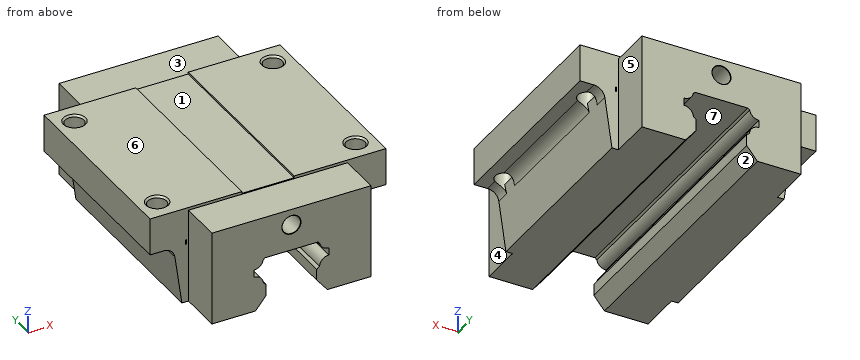
from build123d import *

# Parameters (mm, degrees)
SKIZZE1_W                       = 44
SKIZZE1_H                       = 51.3
AUFSATZ_LINEAR_AUSTRAGEN1_DEPTH = 26
SKIZZE2_W                       = 0.25
SKIZZE2_H                       = 17.25
SCHNITT_LINEAR_AUSTRAGEN1_DEPTH = 64.369472146
SKIZZE3_W                       = 14
SKIZZE3_H                       = 0.5
SCHNITT_LINEAR_AUSTRAGEN2_DEPTH = 64.369472146
SKIZZE4_W                       = 0.25
SKIZZE4_H                       = 17.25
SCHNITT_LINEAR_AUSTRAGEN3_DEPTH = 51.3
SKIZZE5_W                       = 42.5
SKIZZE5_H                       = 25.25
AUFSATZ_LINEAR_AUSTRAGEN2_DEPTH = 11.35
SKIZZE6_W                       = 42.5
SKIZZE6_H                       = 25.25
AUFSATZ_LINEAR_AUSTRAGEN3_DEPTH = 11.35
SKIZZE15_W                      = 9.5
SKIZZE15_H                      = 51.3
AUFSATZ_LINEAR_AUSTRAGEN5_DEPTH = 10
SCHNITT_LINEAR_AUSTRAGEN4_DEPTH = 86.838511171
BOHRUNG1_D                      = 4.917
BOHRUNG1_DEPTH                  = 15
BOHRUNG1_TIP                    = 1.477215832
BOHRUNG2_D                      = 4.917
BOHRUNG2_DEPTH                  = 15
BOHRUNG2_TIP                    = 1.477215832
M6_GEWINDEBOHRUNG1_D            = 5
M6_GEWINDEBOHRUNG1_DEPTH        = 17
M6_GEWINDEBOHRUNG1_TIP          = 1.502151548
FASE1_SIZE                      = 0.483
FASE2_SIZE                      = 0.448979592
FASE3_SIZE                      = 0.0915
FASE4_SIZE                      = 0.448979592
AUFSATZ_LINEAR_START            = -51.3
AUFSATZ_LINEAR_AUSTRAGEN6_DEPTH = 51.3
VERRUNDUNG1_R                   = 3


with BuildPart() as part:
    # Skizze1 → Aufsatz-Linear austragen1 (new body)
    with BuildSketch(Plane(origin=(0, 0, 4), x_dir=(-1, 0, 0), z_dir=(0, 0, -1))):
        Rectangle(SKIZZE1_W, SKIZZE1_H)
    extrude(amount=-AUFSATZ_LINEAR_AUSTRAGEN1_DEPTH)

    # Skizze2 → Schnitt-Linear austragen1 (cut, through all)
    with BuildSketch(Plane.XZ.offset(25.65)):
        with Locations((-21.875, 12.625)):
            Rectangle(SKIZZE2_W, SKIZZE2_H)
    extrude(amount=-SCHNITT_LINEAR_AUSTRAGEN1_DEPTH, mode=Mode.SUBTRACT)

    # Skizze3 → Schnitt-Linear austragen2 (cut, through all)
    with BuildSketch(Plane.XZ.offset(25.65)):
        with Locations((0, 29.75)):
            Rectangle(SKIZZE3_W, SKIZZE3_H)
    extrude(amount=-SCHNITT_LINEAR_AUSTRAGEN2_DEPTH, mode=Mode.SUBTRACT)

    # Skizze4 → Schnitt-Linear austragen3 (cut)
    with BuildSketch(Plane.XZ.offset(25.65)):
        with Locations((21.875, 12.625)):
            Rectangle(SKIZZE4_W, SKIZZE4_H)
    extrude(amount=-SCHNITT_LINEAR_AUSTRAGEN3_DEPTH, mode=Mode.SUBTRACT)

    # Skizze5 → Aufsatz-Linear austragen2 (add)
    with BuildSketch(Plane(origin=(0, 25.65, 0), x_dir=(-1, 0, 0), z_dir=(0, 1, 0))):
        with Locations((0, 16.625)):
            Rectangle(SKIZZE5_W, SKIZZE5_H)
    extrude(amount=AUFSATZ_LINEAR_AUSTRAGEN2_DEPTH)

    # Skizze6 → Aufsatz-Linear austragen3 (add)
    with BuildSketch(Plane.XZ.offset(25.65)):
        with Locations((0, 16.625)):
            Rectangle(SKIZZE6_W, SKIZZE6_H)
    extrude(amount=AUFSATZ_LINEAR_AUSTRAGEN3_DEPTH)

    # Skizze15 → Aufsatz-Linear austragen5 (add)
    with BuildSketch(Plane.XY.offset(30)):
        with Locations((-26.75, 0)):
            Rectangle(SKIZZE15_W, SKIZZE15_H)
        with Locations((26.75, 0)):
            Rectangle(SKIZZE15_W, SKIZZE15_H)
    extrude(amount=-AUFSATZ_LINEAR_AUSTRAGEN5_DEPTH)

    # Skizze7 → Schnitt-Linear austragen4 (cut, through all)
    with BuildSketch(Plane.XZ.offset(37)):
        with BuildLine():
            Line((-9.59375, 4), (9.59375, 4))
            Line((9.59375, 4), (6.75, 7.5))
            Line((6.75, 7.5), (6.75, 10.5))
            Line((6.75, 10.5), (7.5, 11.109375))
            ThreePointArc((7.5, 11.109375), (8.270470592, 12.806156162), (10, 13.5))
            Line((10, 13.5), (10, 15.5))
            ThreePointArc((10, 15.5), (8.232233047, 16.232233047), (7.5, 18))
            Line((7.5, 18), (-7.5, 18))
            ThreePointArc((-7.5, 18), (-8.232233047, 16.232233047), (-10, 15.5))
            Line((-10, 15.5), (-10, 13.5))
            ThreePointArc((-10, 13.5), (-8.270470592, 12.806156162), (-7.5, 11.109375))
            Line((-7.5, 11.109375), (-6.75, 10.5))
            Line((-6.75, 10.5), (-6.75, 7.5))
            Line((-6.75, 7.5), (-9.59375, 4))
        make_face()
    extrude(amount=-SCHNITT_LINEAR_AUSTRAGEN4_DEPTH, mode=Mode.SUBTRACT)

    # Bohrung1
    with Locations(Plane(origin=(0, -37, 0), x_dir=(-1, 0, 0), z_dir=(0, -1, 0))):
        with Locations((0, -25)):
            Hole(BOHRUNG1_D / 2, depth=BOHRUNG1_DEPTH)
            with Locations((0, 0, -(BOHRUNG1_DEPTH + BOHRUNG1_TIP / 2))):  # 118° drill point
                Cone(0, BOHRUNG1_D / 2, BOHRUNG1_TIP, mode=Mode.SUBTRACT)

    # Bohrung2
    with Locations(Plane(origin=(0, 37, 0), x_dir=(1, 0, 0), z_dir=(0, 1, 0))):
        with Locations((0, -25)):
            Hole(BOHRUNG2_D / 2, depth=BOHRUNG2_DEPTH)
            with Locations((0, 0, -(BOHRUNG2_DEPTH + BOHRUNG2_TIP / 2))):  # 118° drill point
                Cone(0, BOHRUNG2_D / 2, BOHRUNG2_TIP, mode=Mode.SUBTRACT)

    # M6 Gewindebohrung1
    with Locations(Plane.XY.offset(30)):
        with Locations((26.5, -20), (26.5, 20), (-26.5, 20), (-26.5, -20)):
            Hole(M6_GEWINDEBOHRUNG1_D / 2, depth=M6_GEWINDEBOHRUNG1_DEPTH)
            with Locations((0, 0, -(M6_GEWINDEBOHRUNG1_DEPTH + M6_GEWINDEBOHRUNG1_TIP / 2))):  # 118° drill point
                Cone(0, M6_GEWINDEBOHRUNG1_D / 2, M6_GEWINDEBOHRUNG1_TIP, mode=Mode.SUBTRACT)

    # Fase1
    fase1_edges = [part.edges().sort_by_distance(p)[0] for p in [
        (-24, -20, 30),
        (-24, 20, 30),
        (29, 20, 30),
        (29, -20, 30),
    ]]
    chamfer(fase1_edges, length=FASE1_SIZE)

    # Fase2
    # the kernel refuses this chamfer: 0.448979592, 0.406117321 mm, written as the material it adds along each edge
    with BuildSketch(Plane(origin=(-7.5, -37, 18), x_dir=(1, 0, 0), z_dir=(0, 1, 0))) as fase2_piece_1:
        with BuildLine():
            Line((FASE2_SIZE, 0), (-0.03932739, 0.441690284))
            ThreePointArc((-0.03932739, 0.441690284), (-0.010448273, 0.22832477), (0, 0))
            Line((0, 0), (FASE2_SIZE, 0))
        make_face()
    extrude(amount=74)

    # Fase3
    fase3_edges = [part.edges().sort_by_distance(p)[0] for p in [
        (-2.4585, -37, 25),
        (2.4585, 37, 25),
    ]]
    chamfer(fase3_edges, length=FASE3_SIZE)

    # Fase4
    # the kernel refuses this chamfer: 0.448979592, 0.406117321 mm, written as the material it adds along each edge
    with BuildSketch(Plane(origin=(7.5, -37, 18), x_dir=(0.08868753028202897, 0, -0.9960594972050988), z_dir=(0, 1, 0))) as fase4_piece_1:
        with BuildLine():
            Line((0.443437651, 0), (-FASE4_SIZE * 0.0886875302498, FASE4_SIZE * 0.996059496843))
            Line((-FASE4_SIZE * 0.0886875302498, FASE4_SIZE * 0.996059496843), (0, 0))
            ThreePointArc((0, 0), (0.228351687, 0.009842458), (0.443437651, 0))
        make_face()
    extrude(amount=74)

    # Skizze16 → Aufsatz-Linear austragen6 (add)
    with BuildSketch(Plane.XZ.offset(25.65).offset(AUFSATZ_LINEAR_START)):
        Polygon((-21.75, 4), (-21.75, 20), (-25.25, 20), (-23, 4), align=None)
        Polygon((21.75, 20), (25.25, 20), (23, 4), (21.75, 4), align=None)
    extrude(amount=AUFSATZ_LINEAR_AUSTRAGEN6_DEPTH)

    # Verrundung1
    # the kernel refuses this fillet: 3 mm, written as the material it adds along each edge
    with BuildSketch(Plane(origin=(-25.25, 25.65, 20), x_dir=(0.13925483139909986, 0, -0.9902565788380344), z_dir=(0, -1, 0))) as verrundung1_piece_1_section:
        with BuildLine():
            CenterArc((VERRUNDUNG1_R * 0.869214289504, -VERRUNDUNG1_R), VERRUNDUNG1_R, 90, 81.995271143)
            Line((-VERRUNDUNG1_R * 0.121042289335, -VERRUNDUNG1_R * 0.860745168601), (0, 0))
            Line((0, 0), (VERRUNDUNG1_R * 0.869214289504, 0))
        make_face()
    verrundung1_piece_1 = extrude(amount=10.004043662, mode=Mode.PRIVATE)
    verrundung1_piece_1 = verrundung1_piece_1 - Plane(origin=(-26.5, 20, 20), x_dir=(-1, 0, 0), z_dir=(0, 0, -1)) * Cylinder(2.5, 31, mode=Mode.PRIVATE)
    add(verrundung1_piece_1)
    with BuildSketch(Plane(origin=(-25.25, 24.354043662, 20), x_dir=(0.13925483139909986, 0, -0.9902565788380344), z_dir=(0, -1, 0))) as verrundung1_piece_2_section:
        with BuildLine():
            CenterArc((VERRUNDUNG1_R * 0.869214289504, -VERRUNDUNG1_R), VERRUNDUNG1_R, 90, 81.995271143)
            Line((-VERRUNDUNG1_R * 0.121042289335, -VERRUNDUNG1_R * 0.860745168601), (0, 0))
            Line((0, 0), (VERRUNDUNG1_R * 0.869214289504, 0))
        make_face()
    verrundung1_piece_2 = extrude(amount=48.708087324, mode=Mode.PRIVATE)
    verrundung1_piece_2 = verrundung1_piece_2 - Plane(origin=(-26.5, -20, 20), x_dir=(-1, 0, 0), z_dir=(0, 0, -1)) * Cylinder(2.5, 108, mode=Mode.PRIVATE)
    verrundung1_piece_2 = verrundung1_piece_2 - Plane(origin=(-26.5, 20, 20), x_dir=(-1, 0, 0), z_dir=(0, 0, -1)) * Cylinder(2.5, 108, mode=Mode.PRIVATE)
    add(verrundung1_piece_2)
    with BuildSketch(Plane(origin=(-25.25, -15.645956338, 20), x_dir=(0.13925483139909986, 0, -0.9902565788380344), z_dir=(0, -1, 0))) as verrundung1_piece_3_section:
        with BuildLine():
            CenterArc((VERRUNDUNG1_R * 0.869214289504, -VERRUNDUNG1_R), VERRUNDUNG1_R, 90, 81.995271143)
            Line((-VERRUNDUNG1_R * 0.121042289335, -VERRUNDUNG1_R * 0.860745168601), (0, 0))
            Line((0, 0), (VERRUNDUNG1_R * 0.869214289504, 0))
        make_face()
    verrundung1_piece_3 = extrude(amount=10.004043662, mode=Mode.PRIVATE)
    verrundung1_piece_3 = verrundung1_piece_3 - Plane(origin=(-26.5, -20, 20), x_dir=(-1, 0, 0), z_dir=(0, 0, -1)) * Cylinder(2.5, 31, mode=Mode.PRIVATE)
    add(verrundung1_piece_3)
    with BuildSketch(Plane(origin=(25.25, 25.65, 20), x_dir=(1, 0, 0), z_dir=(0, -1, 0))) as verrundung1_piece_4_section:
        with BuildLine():
            CenterArc((VERRUNDUNG1_R * 0.869214289504, -VERRUNDUNG1_R), VERRUNDUNG1_R, 90, 81.995271143)
            Line((-VERRUNDUNG1_R * 0.121042289335, -VERRUNDUNG1_R * 0.860745168601), (0, 0))
            Line((0, 0), (VERRUNDUNG1_R * 0.869214289504, 0))
        make_face()
    verrundung1_piece_4 = extrude(amount=10.004043662, mode=Mode.PRIVATE)
    verrundung1_piece_4 = verrundung1_piece_4 - Plane(origin=(26.5, 20, 20), x_dir=(-1, 0, 0), z_dir=(0, 0, -1)) * Cylinder(2.5, 31, mode=Mode.PRIVATE)
    add(verrundung1_piece_4)
    with BuildSketch(Plane(origin=(25.25, 24.354043662, 20), x_dir=(1, 0, 0), z_dir=(0, -1, 0))) as verrundung1_piece_5_section:
        with BuildLine():
            CenterArc((VERRUNDUNG1_R * 0.869214289504, -VERRUNDUNG1_R), VERRUNDUNG1_R, 90, 81.995271143)
            Line((-VERRUNDUNG1_R * 0.121042289335, -VERRUNDUNG1_R * 0.860745168601), (0, 0))
            Line((0, 0), (VERRUNDUNG1_R * 0.869214289504, 0))
        make_face()
    verrundung1_piece_5 = extrude(amount=48.708087324, mode=Mode.PRIVATE)
    verrundung1_piece_5 = verrundung1_piece_5 - Plane(origin=(26.5, -20, 20), x_dir=(-1, 0, 0), z_dir=(0, 0, -1)) * Cylinder(2.5, 108, mode=Mode.PRIVATE)
    verrundung1_piece_5 = verrundung1_piece_5 - Plane(origin=(26.5, 20, 20), x_dir=(-1, 0, 0), z_dir=(0, 0, -1)) * Cylinder(2.5, 108, mode=Mode.PRIVATE)
    add(verrundung1_piece_5)
    with BuildSketch(Plane(origin=(25.25, -15.645956338, 20), x_dir=(1, 0, 0), z_dir=(0, -1, 0))) as verrundung1_piece_6_section:
        with BuildLine():
            CenterArc((VERRUNDUNG1_R * 0.869214289504, -VERRUNDUNG1_R), VERRUNDUNG1_R, 90, 81.995271143)
            Line((-VERRUNDUNG1_R * 0.121042289335, -VERRUNDUNG1_R * 0.860745168601), (0, 0))
            Line((0, 0), (VERRUNDUNG1_R * 0.869214289504, 0))
        make_face()
    verrundung1_piece_6 = extrude(amount=10.004043662, mode=Mode.PRIVATE)
    verrundung1_piece_6 = verrundung1_piece_6 - Plane(origin=(26.5, -20, 20), x_dir=(-1, 0, 0), z_dir=(0, 0, -1)) * Cylinder(2.5, 31, mode=Mode.PRIVATE)
    add(verrundung1_piece_6)


solid = part.part
Source: CAD feature listing. Evaluate the final solid. Frame: model axes, mm. Face numbers are marked on the shaded views. A direction names the side the tool comes from. Coordinates: 2 decimals unless noted, no trailing zeros. Write each loop counter-clockwise with the first axis right and the second up, starting at its lowest first coordinate (ties: lowest second). Pieces come first, ordered by that corner, then holes. Notation, with made-up numbers: M 26,-3.75 L 78,-3.75 A27 ccw 78,15.25 Z; hole C 60.5,29 d4. An arc over 180 degrees is marked long. Use a Markdown table: item, result.
1) First-contact query: pin 1 Ø1 at (y, z) = (2.5, 11.5) entering from +X (3 decimals); pin 2 Ø1.5 at (y, z) = (-2, 9) entering from -X; pin 3 Ø3.5 at (y, z) = (-30.5, 10.5) entering from +X. Flat tips, straight axial feed; report the tip coordinate or a pass-through.
Conclusion:
| item | result |
|---|---|
| pin 1 | stops at x = 24.125 |
| pin 2 | stops at x = -23.81 |
| pin 3 | stops at x = 21.25 |
2) Ray query, L1, parallel to X at y = 7, z = 21; L2, parallel to Y at x = 26.5, z = 27.25; L3, parallel to Z at x = 0, y = 26. Return the intervals inside material, ascending.
Conclusion:
| item | result |
|---|---|
| L1 | x = -31.5 to -22, -21.75 to 21.75, 22 to 31.5 |
| L2 | y = -25.65 to -22.5, -17.5 to 17.5, 22.5 to 25.65 |
| L3 | z = 18 to 22.54, 27.46 to 29.25 |
3) Mould query, pull axis X, two halves, no side actions, for the marked faces 5, 6 and 7. Classes: pulls with the +X half, pulls with the -X half, needs draft (parallel to the pull), parting line crosses it, or undercut.
Conclusion:
| item | result |
|---|---|
| face 5 | pulls with the +X half |
| face 6 | needs draft |
| face 7 | undercut |
4) Section A-A, the plane x = 26.5. Output: boundary loops of the cut face in (y, z).
Conclusion:
| item | result |
|---|---|
| outline | M -25.65,19.68 L -22.5,19.68 L -22.5,29.52 L -22.98,30 L -25.65,30 Z; M -17.5,19.68 L 17.5,19.68 L 17.5,29.52 L 17.02,30 L -17.02,30 L -17.5,29.52 Z; M 22.5,19.68 L 25.65,19.68 L 25.65,30 L 22.98,30 L 22.5,29.52 Z |
5) Section C-C, the plane y = -15.5. Give the number of separate pieces and of enclosed holes in the cut face, then the cut area to 3 significant figures.
Conclusion:
| item | result |
|---|---|
| separate pieces | 1 |
| enclosed holes | 2 |
| area | 1,170 mm^2 |
6) Reachability of the marked faces 1, 2, 3 and 4 from +Z, -Z, +X, -X, +Y, -Y: full face, straight path, thin tool, end or side. Return the list, or none.
Conclusion:
| item | result |
|---|---|
| face 1 | +Z, +Y, -Y |
| face 2 | -Z, +Y, -Y |
| face 3 | +Z, +X, -X, +Y |
| face 4 | +Z, -Z, +X, -Y |
